Verification items for the finished model (mm, model axes). Round coordinates to 2 decimals unless told otherwise and drop trailing zeros. Write each loop counter-clockwise with the first axis right and the second up, starting at its lowest first coordinate (ties: lowest second). Pieces come first, ordered by that corner, then holes. Notation, with made-up numbers: (50, 35) - (68, 35) arc R20 ccw to (68, 68) - close; hole circle Ø2 at (3, 63.25). An arc over 180 degrees is marked (long way). Answer as a JSON object with one key per item and string values. Group by question number.
1) Thickness scan on line 1 (Z direction, x = 13.5, y = -4.25); line 2 (Z direction, x = 81, y = 6.5); line 3 (Z direction, x = 480.5, y = 5.5). Record the ranges inside material, lowest first.
2) Go/stop test with a flat-tipped pin: pin 1 Ø2 at (y, z) = (-2.5, -147) entering from +X. Record where the tip stops, or that it passes through.
3) Section check B-B (y = 3.75). Enter the section's corners in (x, z).
4) Section check A-A (x = -96.5). Enter the section's corners in (y, z).
5) Section check D-D (x = 444). Enter the section's corners in (y, z).
6) Section check C-C (z = -101). Enter the section's corners in (x, y), then the cut area to 3 significant figures.
```python
from build123d import *

# Parameters (mm, degrees)
F1_DEPTH      = 7.9375
F2_W          = 12.6746
F2_H          = 12.6746
F3_DEPTH      = 1143.001
F3_DEPTH_BACK = 1751


# Not quite as in the source:
# - an extrude ends at something that could not be found from the text; its depth is read off the source's solid


with BuildPart() as f1:
    # F0 (on Front) → F1 (new body, symmetric)
    with BuildSketch(Plane.XZ):
        Polygon((242.2783725209, -287.3375), (571.5, -7.9375), (571.5, 7.9375), (-571.5, 7.9375), (-571.5, -7.9375), (-395.523637951, -287.3375), align=None)
        Polygon((-386.7609312492, -271.4625), (-552.7386363636, -7.9375), (546.9659090909, -7.9375), (236.4500559004, -271.4625), align=None, mode=Mode.SUBTRACT)
    extrude(amount=F1_DEPTH, both=True)

    # F2 (on face) → F3 (cut, two sides)
    with BuildSketch(Plane(origin=(-571.5, 0, 0), x_dir=(0, -1, 0), z_dir=(-1, 0, 0))) as f3_sk:
        Rectangle(F2_W, F2_H)
    extrude(amount=-F3_DEPTH, mode=Mode.SUBTRACT)
    extrude(f3_sk.sketch, amount=F3_DEPTH_BACK, mode=Mode.SUBTRACT)


solid = f1.part
```
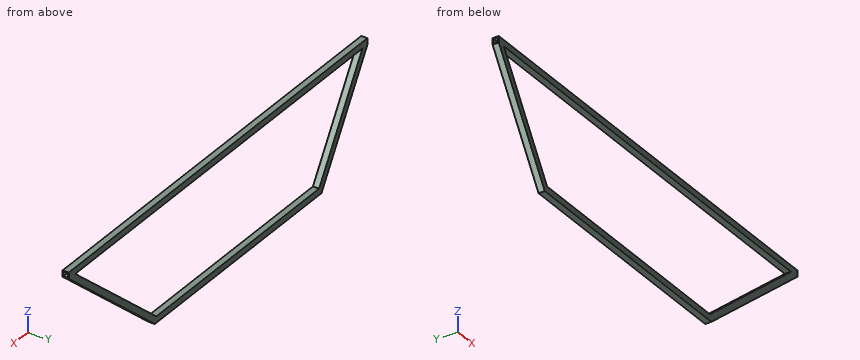
Returned:
{
 "1": {"line 1": "-287.34 to -271.46, -7.94 to -6.34, 6.34 to 7.94", "line 2": "-287.34 to -271.46, -7.94 to 7.94", "line 3": "-85.17 to -64.35, -7.94 to -6.34, 6.34 to 7.94"},
 "2": {"pin 1": "x = 408.82"},
 "3": {"outline": "(-571.5, -7.94) - (-395.52, -287.34) - (242.28, -287.34) - (571.5, -7.94) - (571.5, -6.34) - (-571.5, -6.34) - close; (-571.5, 6.34) - (571.5, 6.34) - (571.5, 7.94) - (-571.5, 7.94) - close; hole (-552.74, -7.94) - (-386.76, -271.46) - (236.45, -271.46) - (546.97, -7.94) - close"},
 "4": {"outline": "(-7.94, -287.34) - (7.94, -287.34) - (7.94, -271.46) - (-7.94, -271.46) - close; (-7.94, -7.94) - (7.94, -7.94) - (7.94, 7.94) - (-7.94, 7.94) - close; hole (-6.34, -6.34) - (6.34, -6.34) - (6.34, 6.34) - (-6.34, 6.34) - close"},
 "5": {"outline": "(-7.94, -116.14) - (7.94, -116.14) - (7.94, -95.32) - (-7.94, -95.32) - close; (-7.94, -7.94) - (7.94, -7.94) - (7.94, 7.94) - (-7.94, 7.94) - close; hole (-6.34, -6.34) - (6.34, -6.34) - (6.34, 6.34) - (-6.34, 6.34) - close"},
 "6": {"outline": "(-512.89, -7.94) - (-494.12, -7.94) - (-494.12, 7.94) - (-512.89, 7.94) - close; (437.31, -7.94) - (461.84, -7.94) - (461.84, 7.94) - (437.31, 7.94) - close", "area": "687 mm2"}
}
